Source: CAD feature listing. Evaluate the final solid. Frame: model axes, mm. Face numbers are marked on the shaded views. A direction names the side the tool comes from. Round coordinates to 2 decimals unless told otherwise and drop trailing zeros. Write each loop counter-clockwise with the first axis right and the second up, starting at its lowest first coordinate (ties: lowest second). Pieces come first, ordered by that corner, then holes. Notation, with made-up numbers: M 32,-37.75 L 56,-37.75 A34 ccw 56,-6.75 Z; hole C 48,-16.5 d2. An arc over 180 degrees is marked long. Use a Markdown table: item, result.
Autodesk Fusion 360 part; units mm, degrees
sketch "Sketch1" plane through (0, 0, 0) normal (0, 1, 0) x (1, 0, 0)
  circle A0 centre (38.1, -38.1) radius 38.1
  circle A1 centre (38.1, -38.1) radius 35.56
  circle A2 centre (38.1, -38.1) radius 3.81
  line L0 (38.1, -38.1) -> (0, -38.1)
  line L1 (38.1, -38.1) -> (76.2, -38.1)
  dimension "d1" = 76.2
  dimension "d2" = 71.12
  dimension "d4" = 7.62
extrude "Extrude1" add sketch "Sketch1" along normal blind 3.81 contours A1 A2 L0 L1 picked at (13.2699, -36.1441) makes body 1
extrude "Extrude2" add sketch "Sketch1" along normal blind 3.81 from surface at 110.49 separate body contours A1 A2 L0 L1 picked at (13.2699, -36.1441) makes body 2
extrude "Extrude3" add sketch "Sketch1" along normal blind 114.3 contours A0 A1 L0 L1 picked at (75.2115, -36.2072) bodies 1 2
sketch "Sketch2" plane through (0, 0, 38.1) normal (0, 0, 1) x (-1, 0, 0)
  line L0 (0, 0) -> (-34.29, 0)
  line L1 (-34.29, 0) -> (-34.29, -3.81)
  line L2 (-34.29, -3.81) -> (-2.54, -3.81)
  line L3 (-2.54, -3.81) -> (-2.54, -110.49)
  line L4 (-2.54, -110.49) -> (-34.29, -110.49)
  line L5 (-34.29, -110.49) -> (-34.29, -114.3)
  line L6 (-34.29, -114.3) -> (0, -114.3)
  line L7 (0, -114.3) -> (0, 0)
  line L8 (0, 0) -> (-7.62, 0)
  line L9 (-7.62, 0) -> (-7.62, -114.3)
  line L10 (-7.62, -114.3) -> (0, -114.3)
  line L11 (0, -114.3) -> (0, 0)
  line L12 (-76.2, 0) -> (-68.58, 0)
  line L13 (-68.58, 0) -> (-68.58, -114.3)
  line L14 (-68.58, -114.3) -> (-76.2, -114.3)
  line L15 (-76.2, -114.3) -> (-76.2, 0)
  dimension "d12" = 7.62
  dimension "d13" = 7.62
extrude "Extrude4" add sketch "Sketch2" against normal blind 27.94 contours L0 L2 L3 L4 L6 L7 L8 L9 L10 L11 | L2 L3 L4 L9 | L12 L13 L14 L15 bodies 1
extrude "Extrude5" cut sketch "Sketch1" along normal blind 121.92 contours A0 A1 L0 L1 | A1 A2 L0 L1 picked at (75.2115, -36.2072) picked at (13.2699, -36.1441) keep common part bodies 1
sketch "Sketch3" plane through (0, 0, 38.1) normal (0, 0, 1) x (-1, 0, 0)
  line L0 (0, 0) -> (-34.29, 0)
  line L1 (-34.29, 0) -> (-34.29, -3.81)
  line L2 (-34.29, -3.81) -> (-7.62, -3.81)
  line L3 (-7.62, -3.81) -> (-7.62, -110.49)
  line L4 (-7.62, -110.49) -> (-34.29, -110.49)
  line L5 (-34.29, -110.49) -> (-34.29, -114.3)
  line L6 (-34.29, -114.3) -> (0, -114.3)
  line L7 (0, -114.3) -> (0, 0)
  circle A0 centre (-3.81, -7.62) radius 2.54
  circle A1 centre (-3.81, -7.62) radius 1.397
  circle A2 centre (-72.39, -7.62) radius 1.397
  circle A3 centre (-72.39, -7.62) radius 2.54
  circle A4 centre (-3.81, -106.68) radius 1.397
  circle A5 centre (-3.81, -106.68) radius 2.54
  circle A6 centre (-72.39, -106.68) radius 1.397
  circle A7 centre (-72.39, -106.68) radius 2.54
  dimension "d18" = 5.08
  dimension "d19" = 7.62
  dimension "d20" = 2.794
  dimension "d23" = -68.58
  dimension "d24" = -99.06
extrude "Extrude6" cut sketch "Sketch3" against normal blind 43.18 contours A1 | A2 | A4 | A6 bodies 1
extrude "Extrude7" cut sketch "Sketch3" against normal blind 25.4 from surface at -2.54 contours A0 | A3 | A5 | A7 bodies 1
sketch "Sketch4" plane through (68.58, 0, 0) normal (-1, 0, 0) x (0, -1, 0)
  line L0 (-3.81, 19.7838) -> (-3.81, 38.1)
  line L1 (-3.81, 38.1) -> (-110.49, 38.1)
  line L2 (-110.49, 38.1) -> (-110.49, 19.7838)
  line L3 (-110.49, 19.7838) -> (-3.81, 19.7838)
  line L4 (-50.8, 38.1) -> (-63.5, 38.1)
  line L5 (-63.5, 38.1) -> (-63.5, 28.575)
  line L6 (-63.5, 28.575) -> (-50.8, 28.575)
  line L7 (-50.8, 28.575) -> (-50.8, 38.1)
  line L8 (0, 38.1) -> (0, 0)
  dimension "d30" = 12.7
  dimension "d31" = 50.8
  dimension "d32" = 9.525
extrude "Extrude8" cut sketch "Sketch4" against normal blind 7.62 contours L1 L4 L5 L6 L7 bodies 1
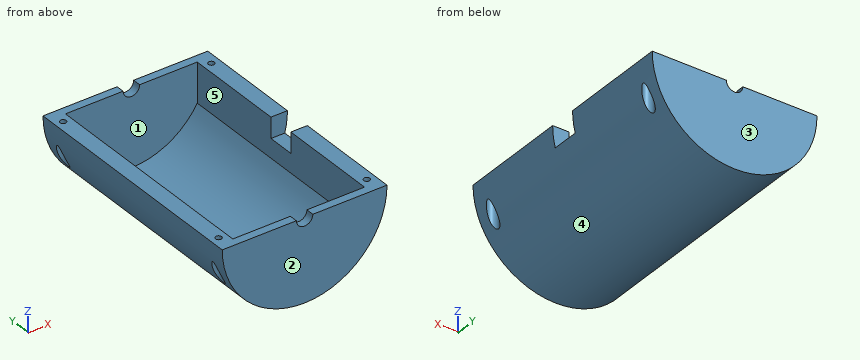
Q1. Reachability of the marked faces 1 and 2 from +Z, -Z, +X, -X, +Y, -Y: full face, straight path, thin tool, end or side. Return the list, or none.
Results are:
| item | result |
|---|---|
| face 1 | +Z |
| face 2 | +Z, -Z, +X, -X, -Y |
Q2. Section D-D on x = 3.81. Return loops of the section in (y, z), plus the area to 3 significant figures.
Results are:
| item | result |
|---|---|
| outline | M 0,21.49 L 5.08,21.49 L 5.08,35.56 L 6.22,35.56 L 6.22,38.1 L 0,38.1 Z; M 9.02,35.56 L 10.16,35.56 L 10.16,21.49 L 104.14,21.49 L 104.14,35.56 L 105.28,35.56 L 105.28,38.1 L 9.02,38.1 Z; M 108.08,35.56 L 109.22,35.56 L 109.22,21.49 L 114.3,21.49 L 114.3,38.1 L 108.08,38.1 Z |
| area | 1,740 mm^2 |
Q3. Section A-A on y = 7.62. Return loops of the section in (x, z), plus the area to 3 significant figures.
Results are:
| item | result |
|---|---|
| outline | M 0,38.1 A38.1 ccw 1.27,28.34 L 1.27,35.56 L 2.41,35.56 L 2.41,38.1 Z; M 5.21,35.56 L 6.35,35.56 L 6.35,17.04 A38.1 ccw 69.85,17.04 L 69.85,35.56 L 70.99,35.56 L 70.99,38.1 L 68.58,38.1 L 68.58,19.78 A35.56 cw 7.62,19.78 L 7.62,38.1 L 5.21,38.1 Z; M 73.79,35.56 L 74.93,35.56 L 74.93,28.34 A38.1 ccw 76.2,38.1 L 73.79,38.1 Z |
| area | 267 mm^2 |
Q4. Line query: L1, parallel to Y at x = 3.81, z = 26.5; L2, parallel to Y at x = 72.39, z = 37.35; L3, parallel to Y at x = 3.81, z = 37.5. Output: solid intervals per line, ascending.
Results are:
| item | result |
|---|---|
| L1 | 0 to 5.08, 10.16 to 104.14, 109.22 to 114.3 |
| L2 | 0 to 6.22, 9.02 to 50.8, 63.5 to 105.28, 108.08 to 114.3 |
| L3 | 0 to 6.22, 9.02 to 105.28, 108.08 to 114.3 |
Q5. Section C-C on x = 38.1. Return loops of the section in (y, z), plus the area to 3 significant figures.
Results are:
| item | result |
|---|---|
| outline | M 0,0 L 114.3,0 L 114.3,34.29 L 110.49,34.29 L 110.49,2.54 L 3.81,2.54 L 3.81,34.29 L 0,34.29 Z |
| area | 532 mm^2 |
Q6. First-contact query: pin 1 Ø1 at (y, z) = (83.5, 21.5) entering from -X; pin 2 Ø4 at (x, y) = (47, 41.5) entering from +Z; pin 3 Ø4.5 at (x, y) = (3.81, 106.68) entering from -Z; pin 4 Ø1.5 at (x, y) = (3.5, 7.5) entering from -Z. Flat tips, straight axial feed; report the tip coordinate or a pass-through.
Results are:
| item | result |
|---|---|
| pin 1 | x = 3.57 |
| pin 2 | z = 4.25 |
| pin 3 | z = 35.56 |
| pin 4 | through |
Q7. Mould query, pull axis X, two halves, no side actions, for the marked faces 3, 4 and 5. Classes: +X half, -X half, draft (parallel to the pull), parting line (faces both ways), or undercut.
Results are:
| item | result |
|---|---|
| face 3 | draft |
| face 4 | parting line |
| face 5 | undercut |
Q8. Section B-B on z = 24. Return loops of the section in (x, y), plus the area to 3 significant figures.
Results are:
| item | result |
|---|---|
| outline | M 2.71,0 L 73.49,0 L 73.49,5.33 A2.54 cw long 73.49,9.91 L 73.49,104.39 A2.54 cw long 73.49,108.97 L 73.49,114.3 L 2.71,114.3 L 2.71,108.97 A2.54 cw long 2.71,104.39 L 2.71,9.91 A2.54 cw long 2.71,5.33 Z; hole M 7.62,3.81 L 68.58,3.81 L 68.58,110.49 L 7.62,110.49 Z |
| area | 1,530 mm^2 |
